Geometry: see drawing. Coordinates: mm, zero at the bounding-box minimum. A direction names the side the tool comes from. Round coordinates to 2 decimals unless told otherwise and drop trailing zeros. Loops run counter-clockwise (first coordinate to the right, second up) from the corner with the lowest first, then second, coordinate; pieces in that order, holes last. Notation, with made-up numbers: (47.5, -30.5) - (70.5, -30.5) arc R27 ccw to (70.5, -1.5) - close; hole circle Ø5 at (42, 25.5). An arc over 180 degrees is marked (long way). Write item = value, one per line. Start each with the question number.
Item 1: Access query for the marked faces 1 and 2. Directions: +Z, -Z, +X, -X, +Y, -Y. A direction counts if a zero-diameter tool reaches every point of the face in a straight line with its end or side. Return the directions, or none.
Item 2: Section C-C (z = 2.5). Return loops of the section in (x, y).
Item 3: First-contact query: pin 1 (4 mm diameter, centred on y = 34, z = 4.5, fed in from -X); pin 2 (2.5 mm diameter, centred on x = 4.5, y = 4.5, fed in from -Z); pin 3 (3.5 mm diameter, centred on y = 2, z = 7, fed in from -X); pin 4 (2 mm diameter, centred on x = 20, z = 9, fed in from -Y). Flat tips, straight axial feed; report the tip coordinate or a pass-through.
Item 4: Section A-A (x = 8). Return loops of the section in (y, z).
Item 5: Line query: line 1 (X direction, y = 20, z = 6); line 2 (X direction, y = 6, z = 6); line 3 (Y direction, x = 35.5, z = 3.75). Output: solid intervals per line, ascending. Write a range as from..to.
Item 6: Section B-B (y = 4.5). Return loops of the section in (x, z).
Item 7: Section D-D (y = 35.5). Return loops of the section in (x, z).
Item 8: Draft query along Y for the marked faces 3, 4 and 5. Return one class per face: pulls with the +Y half, pulls with the -Y half, needs draft (parallel to the pull), parting line crosses it, or undercut.
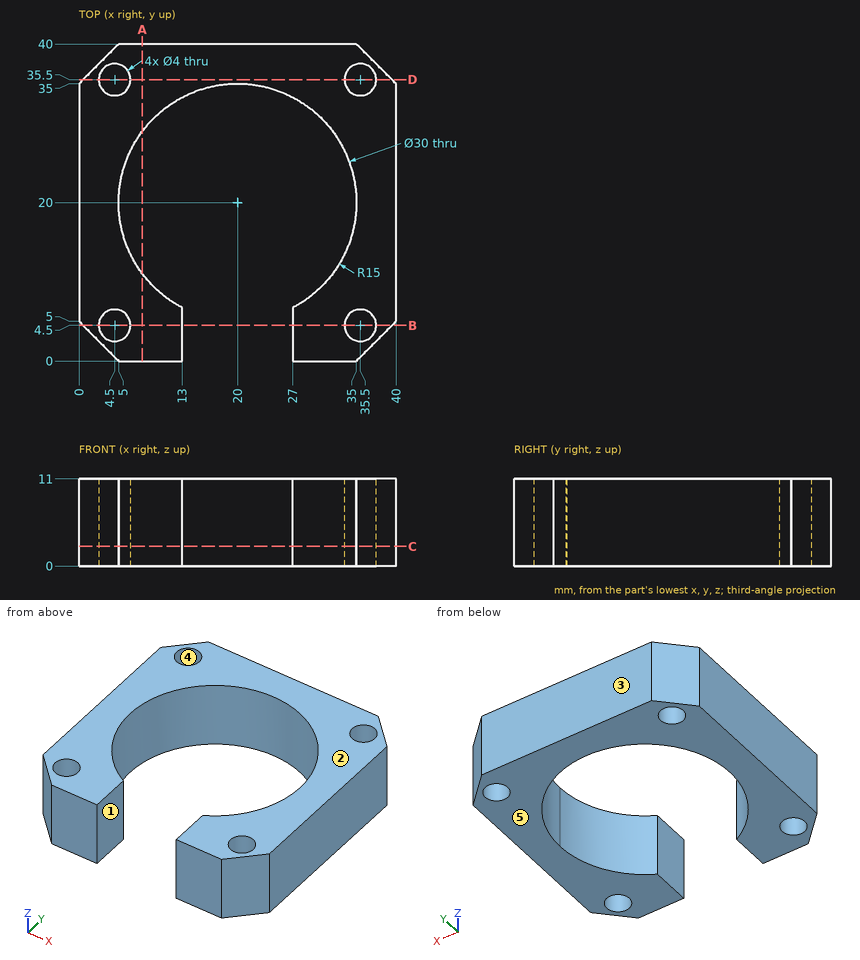
Taken from the geometry:
q1.face_1 = +Z, -Z, -Y
q1.face_2 = +Z, +X, -X, +Y, -Y
q2.outline = (0, 5) - (5, 0) - (13, 0) - (13, 6.73) arc R15 cw (long way) to (35, 20) arc R15 cw to (27, 6.73) - (27, 0) - (35, 0) - (40, 5) - (40, 35) - (35, 40) - (5, 40) - (0, 35) - close; hole circle Ø4 at (4.5, 4.5); hole circle Ø4 at (4.5, 35.5); hole circle Ø4 at (35.5, 4.5); hole circle Ø4 at (35.5, 35.5)
q3.pin_1 = 0
q3.pin_2 = through
q3.pin_3 = 1.25
q3.pin_4 = 34.97
q4.outline = (0, 0) - (11, 0) - (11, 11) - (0, 11) - close; (29, 0) - (40, 0) - (40, 11) - (29, 11) - close
q5.line_1 = 0..5, 35..40
q5.line_2 = 0..3.18, 5.82..13, 27..34.18, 36.82..40
q5.line_3 = 0.5..2.5, 6.5..33.5, 37.5..39.5
q6.outline = (0.5, 0) - (2.5, 0) - (2.5, 11) - (0.5, 11) - close; (6.5, 0) - (13, 0) - (13, 11) - (6.5, 11) - close; (27, 0) - (33.5, 0) - (33.5, 11) - (27, 11) - close; (37.5, 0) - (39.5, 0) - (39.5, 11) - (37.5, 11) - close
q7.outline = (0.5, 0) - (2.5, 0) - (2.5, 11) - (0.5, 11) - close; (6.5, 0) - (33.5, 0) - (33.5, 11) - (6.5, 11) - close; (37.5, 0) - (39.5, 0) - (39.5, 11) - (37.5, 11) - close
q8.face_3 = pulls with the +Y half
q8.face_4 = undercut
q8.face_5 = needs draft
